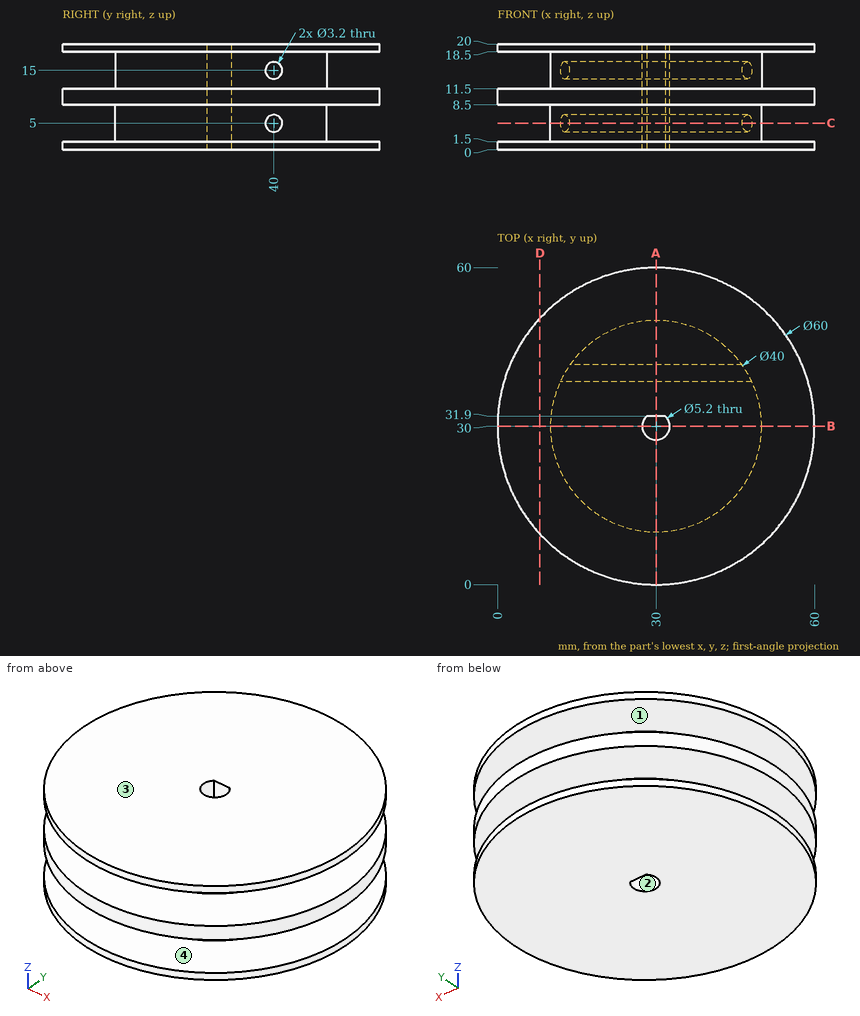
Answer from the drawing. Dimensions are ordinates in mm from the lowest x, y and z of the part. A direction names the side the tool comes from. Round coordinates to 2 decimals unless told otherwise and drop trailing zeros. Write each loop counter-clockwise with the first axis right and the second up, starting at its lowest first coordinate (ties: lowest second). Pieces come first, ordered by that corner, then holes. Notation, with made-up numbers: M -10.5,-35 L 8.5,-35 A27 cw 8.5,-11 Z; hole C -14.5,-10 d4. An arc over 180 degrees is marked long. Write each question's results on one line, items separated by ' | '. Start each with the question number.
Item 1: Straight lines are drawn through the part: L1, parallel to Z at x = 51, y = 41; L2, parallel to Z at x = 29, y = 40; L3, parallel to Y at x = 30, z = 15. For each, find the intervals that lie inside material, in ascending order. Write a range as [from, to].
Item 2: A cutting plane is placed at A-A on x = 30. Write down the section's boundary in (y, z), and give its area (3 significant figures).
Item 3: Flat-ended cylindrical pins translate along their axes: pin 1 Ø5 at (y, z) = (40, 5) entering from +X; pin 2 Ø4 at (x, y) = (44.5, 39.5) entering from -Z; pin 3 Ø4 at (x, z) = (30.5, 14.5) entering from -Y; pin 4 Ø2 at (x, z) = (16, 6.5) entering from -Y. Find the tip coordinate at first contact, or state that the pin passes through.
Item 4: A cutting plane is placed at B-B on y = 30. Write down the section's boundary in (x, z).
Item 5: A cutting plane is placed at D-D on x = 8. Write down the section's boundary in (y, z).
Item 6: A cutting plane is placed at C-C on z = 5. Write down the section's boundary in (x, y).
Item 7: For a pull along Y with two mould halves and no side action, classify the marked faces 1 and 2 as pulls with the +Y half, pulls with the -Y half, needs draft (parallel to the pull), parting line crosses it, or undercut.
Item 8: For the marked faces 3 and 4, determine the directions among +Z, -Z, +X, -X, +Y, -Y from which every point of the face is accessible in a straight line to the end or side of a thin tool.
Check sheet entries:
1) L1: [0, 1.5], [8.5, 11.5], [18.5, 20] | L2: [0, 3.4], [6.6, 13.4], [16.6, 20] | L3: [10, 27.4], [31.9, 38.4], [41.6, 50]
2) outline: M 0,0 L 27.4,0 L 27.4,20 L 0,20 L 0,18.5 L 10,18.5 L 10,11.5 L 0,11.5 L 0,8.5 L 10,8.5 L 10,1.5 L 0,1.5 Z; M 31.9,0 L 60,0 L 60,1.5 L 50,1.5 L 50,8.5 L 60,8.5 L 60,11.5 L 50,11.5 L 50,18.5 L 60,18.5 L 60,20 L 31.9,20 Z; hole C 40,5 d3.2; hole C 40,15 d3.2 | area: 814 mm²
3) pin 1: x = 48.54 | pin 2: z = 0 | pin 3: y = 10 | pin 4: y = 14.8
4) outline: M 0,0 L 27.4,0 L 27.4,20 L 0,20 L 0,18.5 L 10,18.5 L 10,11.5 L 0,11.5 L 0,8.5 L 10,8.5 L 10,1.5 L 0,1.5 Z; M 32.6,0 L 60,0 L 60,1.5 L 50,1.5 L 50,8.5 L 60,8.5 L 60,11.5 L 50,11.5 L 50,18.5 L 60,18.5 L 60,20 L 32.6,20 Z
5) outline: M 9.6,0 L 50.4,0 L 50.4,1.5 L 9.6,1.5 Z; M 9.6,8.5 L 50.4,8.5 L 50.4,11.5 L 9.6,11.5 Z; M 9.6,18.5 L 50.4,18.5 L 50.4,20 L 9.6,20 Z
6) outline: M 11.85,38.4 A20 ccw long 48.15,38.4 Z; M 13.71,41.6 L 46.29,41.6 A20 ccw Z; hole M 28.23,31.9 A2.6 ccw long 31.77,31.9 Z
7) face 1: needs draft | face 2: undercut
8) face 3: +Z, +X, -X, +Y, -Y | face 4: none
